```python
from build123d import *

# Parameters (mm, degrees)
SKETCH4_W           = 110
SKETCH4_H           = 230
BOSS_EXTRUDE3_DEPTH = 80
SKETCH5_W           = 106
SKETCH5_H           = 113
CUT_EXTRUDE2_DEPTH  = 79.8
SKETCH6_R           = 2.5
CUT_EXTRUDE3_DEPTH  = 130


with BuildPart() as part:
    # Sketch4 → Boss-Extrude3 (new body)
    with BuildSketch(Plane(origin=(0, 0, 0), x_dir=(1, 0, 0), z_dir=(0, 1, 0))):
        with Locations((117.5995229, 83.46665824)):
            Rectangle(SKETCH4_W, SKETCH4_H)
    extrude(amount=BOSS_EXTRUDE3_DEPTH)

    # Sketch5 → Cut-Extrude2 (cut)
    with BuildSketch(Plane(origin=(0, 80, 0), x_dir=(1, 0, 0), z_dir=(0, 1, 0))):
        with Locations((117.5995229, 139.96665824)):
            Rectangle(SKETCH5_W, SKETCH5_H)
        with Locations((117.5995229, 26.96665824)):
            Rectangle(SKETCH5_W, SKETCH5_H)
    extrude(amount=-CUT_EXTRUDE2_DEPTH, mode=Mode.SUBTRACT)

    # Sketch6 → Cut-Extrude3 (cut)
    with BuildSketch(Plane.ZY.offset(-62.5995229)):
        with Locations((-158.46665824, 70)):
            Circle(SKETCH6_R)
        with Locations((-8.46665824, 70)):
            Circle(SKETCH6_R)
    extrude(amount=-CUT_EXTRUDE3_DEPTH, mode=Mode.SUBTRACT)


solid = part.part
```
Verification items for the finished model (mm, model axes). A direction names the side the tool comes from. Coordinates: 2 decimals unless noted, no trailing zeros. Write each loop counter-clockwise with the first axis right and the second up, starting at its lowest first coordinate (ties: lowest second). Pieces come first, ordered by that corner, then holes. Notation, with made-up numbers: (68.25, -32.5) - (114.25, -32.5) arc R22 ccw to (114.25, -5.5) - close; hole circle Ø6 at (-27.5, 50). An arc over 180 degrees is marked (long way). Write item = value, one per line.
Q1. Mould release check, pull along Y, two halves, no side actions. Record for faces 3 (the face through (64, 80, -84)), 4 (the face through (63.59, 67.56, -9.01)), 5 (the face through (117, 39, -198.467)): released by +Y, released by -Y, zero draft, split by the parting line, or undercut.
Answer:
face_3 = released by +Y
face_4 = undercut
face_5 = zero draft
Q2. Go/stop test with flat-tipped pins: pin 1 Ø10 at (x, z) = (109.5, -44) entering from +Y; pin 2 Ø3 at (y, z) = (70, -158.47) entering from -X. Record where each tip stops, or that it passes through.
Answer:
pin_1 = 0.2
pin_2 = through
Q3. Access from +Z, -Z, +X, -X, +Y, -Y to the whole of each face (thin tool, end or side, straight path). Record for faces 1 (the face through (117, 0.2, -85)), 2 (the face through (117, 39, 31.533)).
Answer:
face_1 = +Y
face_2 = +Z, +X, -X, +Y, -Y
Q4. Cross-section at A-A (y = 70). Enter the section's corners in (x, z), plus the area to 3 significant figures.
Answer:
outline = (62.6, -198.47) - (172.6, -198.47) - (172.6, -160.97) - (170.6, -160.97) - (170.6, -196.47) - (64.6, -196.47) - (64.6, -160.97) - (62.6, -160.97) - close; (62.6, -155.97) - (64.6, -155.97) - (64.6, -10.97) - (62.6, -10.97) - close; (62.6, -5.97) - (64.6, -5.97) - (64.6, 29.53) - (170.6, 29.53) - (170.6, -5.97) - (172.6, -5.97) - (172.6, 31.53) - (62.6, 31.53) - close; (170.6, -155.97) - (172.6, -155.97) - (172.6, -10.97) - (170.6, -10.97) - close
area = 1,300 mm²
Q5. Cross-section at B-B (y = 52.5). Enter the section's corners in (x, z), plus the area to 3 significant figures.
Answer:
outline = (62.6, -198.47) - (172.6, -198.47) - (172.6, 31.53) - (62.6, 31.53) - close; hole (64.6, -196.47) - (170.6, -196.47) - (170.6, 29.53) - (64.6, 29.53) - close
area = 1,340 mm²
Q6. Material ranges on L1, parallel to X at y = 24.5, z = -26; L2, parallel to Z at x = 135.5, y = 55.5; L3, parallel to Y at x = 161, z = -157, recorded low to high. Write a range as from..to.
Answer:
L1 = 62.6..64.6, 170.6..172.6
L2 = -198.47..-196.47, 29.53..31.53
L3 = 0..0.2
Q7. Cross-section at C-C (x = 98). Enter the section's corners in (y, z), plus the area to 3 significant figures.
Answer:
outline = (0, -198.47) - (80, -198.47) - (80, -196.47) - (0.2, -196.47) - (0.2, 29.53) - (80, 29.53) - (80, 31.53) - (0, 31.53) - close
area = 365 mm²
Q8. Cross-section at D-D (z = -79). Enter the section's corners in (x, y).
Answer:
outline = (62.6, 0) - (172.6, 0) - (172.6, 80) - (170.6, 80) - (170.6, 0.2) - (64.6, 0.2) - (64.6, 80) - (62.6, 80) - close
